```python
from build123d import *

# Parameters (mm, degrees)
SKETCH1_R               = 2
BOSS_EXTRUDE4_DEPTH     = 34.75
SKETCH5_R               = 2
CUT_EXTRUDE2_DEPTH      = 22.75
CUT_EXTRUDE3_REACH      = 59.871
CUT_EXTRUDE4_DEPTH      = 63.586120666
CUT_EXTRUDE5_REACH      = 61.819
CUT_EXTRUDE5_END_RADIUS = 37.906002519
SKETCH10_R              = 1.8
CUT_EXTRUDE6_REACH      = 59.074
SKETCH11_RX             = 1.8
SKETCH11_RY             = 1.799979565
CUT_EXTRUDE7_REACH      = 59.075
SKETCH11_4_RX           = 1.8
SKETCH11_4_RY           = 1.799979565
CUT_EXTRUDE8_DEPTH      = 9.85
SKETCH15_R              = 2
CUT_EXTRUDE9_DEPTH      = 2.38
SKETCH16_R              = 1.25
CUT_EXTRUDE10_DEPTH     = 6.1
SKETCH17_W              = 2.2
SKETCH17_H              = 4.33
CUT_EXTRUDE11_DEPTH     = 6.55
BOSS_EXTRUDE5_DEPTH     = 2.2
BOSS_EXTRUDE6_DEPTH     = 2.2


with BuildPart() as part:
    # Sketch1 → Boss-Extrude4 (new body)
    with BuildSketch(Plane.XY):
        with BuildLine():
            Line((-25.9, -19.75), (-11.5, -19.75))
            ThreePointArc((-11.5, -19.75), (-8.671572875, -18.578427125), (-7.5, -15.75))
            Line((-7.5, -15.75), (-7.5, -13))
            ThreePointArc((-7.5, -13), (0, -5.5), (7.5, -13))
            Line((7.5, -13), (7.5, -15.75))
            ThreePointArc((7.5, -15.75), (8.671572875, -18.578427125), (11.5, -19.75))
            Line((11.5, -19.75), (25.9, -19.75))
            ThreePointArc((25.9, -19.75), (31.556854249, -17.406854249), (33.9, -11.75))
            Line((33.9, -11.75), (33.9, 11.75))
            ThreePointArc((33.9, 11.75), (31.556854249, 17.406854249), (25.9, 19.75))
            Line((25.9, 19.75), (14.643684646, 19.75))
            ThreePointArc((14.643684646, 19.75), (0, 31.5), (-14.643684646, 19.75))
            Line((-14.643684646, 19.75), (-25.9, 19.75))
            ThreePointArc((-25.9, 19.75), (-31.556854249, 17.406854249), (-33.9, 11.75))
            Line((-33.9, 11.75), (-33.9, -11.75))
            ThreePointArc((-33.9, -11.75), (-31.556854249, -17.406854249), (-25.9, -19.75))
        make_face()
        with Locations((-15.9, 10.944699181)):
            Circle(SKETCH1_R, mode=Mode.SUBTRACT)
        with Locations(Location((-15.9, -10.944699181, 0), (0, 0, 180))):
            Circle(SKETCH1_R, mode=Mode.SUBTRACT)
        with Locations((15.9, -10.944699181)):
            Circle(SKETCH1_R, mode=Mode.SUBTRACT)
        with Locations(Location((15.9, 10.944699181, 0), (0, 0, 180))):
            Circle(SKETCH1_R, mode=Mode.SUBTRACT)
    extrude(amount=BOSS_EXTRUDE4_DEPTH)

    # Sketch5 → Cut-Extrude2 (cut)
    with BuildSketch(Plane.XY.offset(34.75)):
        with BuildLine():
            Line((33.9, -11.75), (33.9, 11.75))
            ThreePointArc((33.9, 11.75), (31.556854249, 17.406854249), (25.9, 19.75))
            Line((25.9, 19.75), (14.643684646, 19.75))
            ThreePointArc((14.643684646, 19.75), (0, 31.5), (-14.643684646, 19.75))
            Line((-14.643684646, 19.75), (-25.9, 19.75))
            ThreePointArc((-25.9, 19.75), (-31.556854249, 17.406854249), (-33.9, 11.75))
            Line((-33.9, 11.75), (-33.9, -11.75))
            ThreePointArc((-33.9, -11.75), (-31.556854249, -17.406854249), (-25.9, -19.75))
            Line((-25.9, -19.75), (-11.5, -19.75))
            ThreePointArc((-11.5, -19.75), (-8.671572875, -18.578427125), (-7.5, -15.75))
            Line((-7.5, -15.75), (-7.5, -13))
            ThreePointArc((-7.5, -13), (0, -5.5), (7.5, -13))
            Line((7.5, -13), (7.5, -15.75))
            ThreePointArc((7.5, -15.75), (8.671572875, -18.578427125), (11.5, -19.75))
            Line((11.5, -19.75), (25.9, -19.75))
            ThreePointArc((25.9, -19.75), (31.556854249, -17.406854249), (33.9, -11.75))
        make_face()
        with Locations((-15.9, 10.944699181)):
            Circle(SKETCH5_R, mode=Mode.SUBTRACT)
        with BuildLine():
            Line((-23.3, -3.45), (-23.3, 2.199999619))
            ThreePointArc((-23.3, 2.199999619), (0.199916465, 10.363760615), (23.699998093, 2.200475068))
            Line((23.699998093, 2.200475068), (23.699998093, -3.45))
            Line((23.699998093, -3.45), (-23.3, -3.45))
        make_face(mode=Mode.SUBTRACT)
    extrude(amount=-CUT_EXTRUDE2_DEPTH, mode=Mode.SUBTRACT)

    # Sketch6 → Cut-Extrude3 (cut, up to next)
    with BuildSketch(Plane.XY.offset(34.75), mode=Mode.PRIVATE) as cut_extrude3_sk1:
        with BuildLine():
            Line((-5.499999046, 14.493093188), (-5.499999046, 17.489830849))
            ThreePointArc((-5.499999046, 17.489830849), (0, 22.989829895), (5.499999046, 17.489830849))
            Line((5.499999046, 17.489830849), (5.499999046, 14.493093188))
            ThreePointArc((5.499999046, 14.493093188), (0, 8.993094142), (-5.499999046, 14.493093188))
        make_face()
    cut_extrude3_tool1 = extrude(cut_extrude3_sk1.sketch, amount=-CUT_EXTRUDE3_REACH, mode=Mode.PRIVATE) & part.part
    add(cut_extrude3_tool1.solids().sort_by_distance((0, 15.991462, 34.75))[0], mode=Mode.SUBTRACT)

    # Sketch9 → Cut-Extrude4 (cut, through all)
    with BuildSketch(Plane(origin=(0, 19.75, 0), x_dir=(1, 0, 0), z_dir=(0, 1, 0))):
        Polygon((-29.366805248, 0), (-26.65, -3.88), (-22.86, -3.88), (-20.143194752, 0), align=None)
        Polygon((22.86, -3.88), (20.143194752, 0), (29.366805248, 0), (26.65, -3.88), align=None)
    extrude(amount=-CUT_EXTRUDE4_DEPTH, mode=Mode.SUBTRACT)

    # Cut-Extrude5: up to this cylinder (the profile starts inside it)
    cut_extrude5_end = Plane(origin=(0.20029992, -27.542241902, 29.5), z_dir=(0, 0, 1)) * Cylinder(CUT_EXTRUDE5_END_RADIUS, 200.450005039, mode=Mode.PRIVATE)
    # Sketch10 → Cut-Extrude5 (cut, up to the surface)
    with BuildSketch(Plane.XZ.offset(3.45), mode=Mode.PRIVATE) as cut_extrude5_sk1:
        with Locations((-17.3, 29.5)):
            Circle(SKETCH10_R)
    cut_extrude5_tool1 = extrude(cut_extrude5_sk1.sketch, amount=-CUT_EXTRUDE5_REACH, mode=Mode.PRIVATE) & cut_extrude5_end
    add(cut_extrude5_tool1.solids().sort_by_distance((-17.3, -3.45, 29.5))[0], mode=Mode.SUBTRACT)
    # Sketch10 → Cut-Extrude5 (cut, up to the surface)
    with BuildSketch(Plane.XZ.offset(3.45), mode=Mode.PRIVATE) as cut_extrude5_sk2:
        with Locations((17.3, 29.5)):
            Circle(SKETCH10_R)
    cut_extrude5_tool2 = extrude(cut_extrude5_sk2.sketch, amount=-CUT_EXTRUDE5_REACH, mode=Mode.PRIVATE) & cut_extrude5_end
    add(cut_extrude5_tool2.solids().sort_by_distance((17.3, -3.45, 29.5))[0], mode=Mode.SUBTRACT)

    # Cut-Extrude6: up to this plane
    cut_extrude6_end = Plane(origin=(0, -1.1, 12), z_dir=(0, 1, 0))
    # Sketch11 → Cut-Extrude6 (cut, up to the surface)
    with BuildSketch(Plane(origin=(-0.04863224, 10.206057531, 0), x_dir=(-0.999988647405363, -0.004764982727443531, 0), z_dir=(0.00476498272744353, -0.9999886474053629, 0)), mode=Mode.PRIVATE) as cut_extrude6_sk1:
        Polygon((13.863688181, -29.5), (15.589965486, -32.49), (19.042520095, -32.49), (20.7687974, -29.5), (19.042520095, -26.51), (15.589965486, -26.51), align=None)
        with Locations(Location((17.316242791, -29.5), (0, 0, -90))):
            Ellipse(SKETCH11_RX, SKETCH11_RY, mode=Mode.SUBTRACT)
    cut_extrude6_tool1 = split(extrude(cut_extrude6_sk1.sketch, amount=CUT_EXTRUDE6_REACH, mode=Mode.PRIVATE), bisect_by=cut_extrude6_end, keep=Keep.BOTH, mode=Mode.PRIVATE)
    add(cut_extrude6_tool1.solids().sort_by_distance((-14.854399, 10.135508, 30.949327))[0], mode=Mode.SUBTRACT)
    # Sketch11 → Cut-Extrude6 (cut, up to the surface)
    with BuildSketch(Plane(origin=(-0.04863224, 10.206057531, 0), x_dir=(-0.999988647405363, -0.004764982727443531, 0), z_dir=(0.00476498272744353, -0.9999886474053629, 0)), mode=Mode.PRIVATE) as cut_extrude6_sk2:
        with Locations(Location((17.316242791, -29.5), (0, 0, -90))):
            Ellipse(SKETCH11_RX, SKETCH11_RY)
    cut_extrude6_tool2 = split(extrude(cut_extrude6_sk2.sketch, amount=CUT_EXTRUDE6_REACH, mode=Mode.PRIVATE), bisect_by=cut_extrude6_end, keep=Keep.BOTH, mode=Mode.PRIVATE)
    add(cut_extrude6_tool2.solids().sort_by_distance((-17.364678, 10.123546, 29.5))[0], mode=Mode.SUBTRACT)

    # Cut-Extrude7: up to this plane
    cut_extrude7_end = Plane(origin=(0, -1.1, 12), z_dir=(0, 1, 0))
    # Sketch11<4> → Cut-Extrude7 (cut, up to the surface)
    with BuildSketch(Plane(origin=(-0.04863224, 10.206057531, 0), x_dir=(-0.999988647405363, -0.004764982727443531, 0), z_dir=(0.00476498272744353, -0.9999886474053629, 0)), mode=Mode.PRIVATE) as cut_extrude7_sk1:
        Polygon((-13.8308098, -29.5), (-15.557087105, -26.51), (-19.009641715, -26.51), (-20.735919019, -29.5), (-19.009641715, -32.49), (-15.557087105, -32.49), align=None)
        with Locations(Location((-17.28336441, -29.5), (0, 0, -90))):
            Ellipse(SKETCH11_4_RX, SKETCH11_4_RY, mode=Mode.SUBTRACT)
    cut_extrude7_tool1 = split(extrude(cut_extrude7_sk1.sketch, amount=CUT_EXTRUDE7_REACH, dir=(0, -1, 0), mode=Mode.PRIVATE), bisect_by=cut_extrude7_end, keep=Keep.BOTH, mode=Mode.PRIVATE)
    add(cut_extrude7_tool1.solids().sort_by_distance((14.724256, 10.276451, 28.050673))[0], mode=Mode.SUBTRACT)
    # Sketch11<4> → Cut-Extrude7 (cut, up to the surface)
    with BuildSketch(Plane(origin=(-0.04863224, 10.206057531, 0), x_dir=(-0.999988647405363, -0.004764982727443531, 0), z_dir=(0.00476498272744353, -0.9999886474053629, 0)), mode=Mode.PRIVATE) as cut_extrude7_sk2:
        with Locations(Location((-17.28336441, -29.5), (0, 0, -90))):
            Ellipse(SKETCH11_4_RX, SKETCH11_4_RY)
    cut_extrude7_tool2 = split(extrude(cut_extrude7_sk2.sketch, amount=CUT_EXTRUDE7_REACH, dir=(0, -1, 0), mode=Mode.PRIVATE), bisect_by=cut_extrude7_end, keep=Keep.BOTH, mode=Mode.PRIVATE)
    add(cut_extrude7_tool2.solids().sort_by_distance((17.234536, 10.288412, 29.5))[0], mode=Mode.SUBTRACT)

    # Sketch14 → Cut-Extrude8 (cut)
    with BuildSketch(Plane(origin=(0, 0, 0), x_dir=(-1, 0, 0), z_dir=(0, 0, -1))):
        Polygon((0, 3), (9.959292144, 8.75), (9.959292144, 23.25), (0, 29), (-9.959292144, 23.25), (-9.959292144, 8.75), align=None)
    extrude(amount=-CUT_EXTRUDE8_DEPTH, mode=Mode.SUBTRACT)

    # Sketch15 → Cut-Extrude9 (cut)
    with BuildSketch(Plane.XY.offset(12)):
        Polygon((-14.167949192, 7.944699181), (-12.435898385, 10.944699181), (-14.167949192, 13.944699181), (-17.632050808, 13.944699181), (-19.364101615, 10.944699181), (-17.632050808, 7.944699181), align=None)
        with Locations((-15.9, 10.944699181)):
            Circle(SKETCH15_R, mode=Mode.SUBTRACT)
        with Locations((-15.9, 10.944699181)):
            Circle(SKETCH15_R)
        Polygon((14.167949192, 13.944699181), (17.632050808, 13.944699181), (19.364101615, 10.944699181), (17.632050808, 7.944699181), (14.167949192, 7.944699181), (12.435898385, 10.944699181), align=None)
        with Locations(Location((15.9, 10.944699181, 0), (0, 0, 180))):
            Circle(SKETCH15_R, mode=Mode.SUBTRACT)
        with Locations(Location((15.9, 10.944699181, 0), (0, 0, 180))):
            Circle(SKETCH15_R)
        Polygon((12.435898385, -10.944699181), (14.167949192, -13.944699181), (17.632050808, -13.944699181), (19.364101615, -10.944699181), (17.632050808, -7.944699181), (14.167949192, -7.944699181), align=None)
        with Locations((15.9, -10.944699181)):
            Circle(SKETCH15_R, mode=Mode.SUBTRACT)
        with Locations((15.9, -10.944699181)):
            Circle(SKETCH15_R)
        Polygon((-17.632050808, -13.944699181), (-19.364101615, -10.944699181), (-17.632050808, -7.944699181), (-14.167949192, -7.944699181), (-12.435898385, -10.944699181), (-14.167949192, -13.944699181), align=None)
        with Locations(Location((-15.9, -10.944699181, 0), (0, 0, 180))):
            Circle(SKETCH15_R, mode=Mode.SUBTRACT)
        with Locations(Location((-15.9, -10.944699181, 0), (0, 0, 180))):
            Circle(SKETCH15_R)
    extrude(amount=-CUT_EXTRUDE9_DEPTH, mode=Mode.SUBTRACT)

    # Sketch16 → Cut-Extrude10 (cut)
    with BuildSketch(Plane.ZY.offset(33.9)):
        with Locations((8.05, 1.13)):
            Circle(SKETCH16_R)
        with Locations((8.05, -8.33)):
            Circle(SKETCH16_R)
    extrude(amount=-CUT_EXTRUDE10_DEPTH, mode=Mode.SUBTRACT)

    # Sketch17 → Cut-Extrude11 (cut)
    with BuildSketch(Plane.XY.offset(12)):
        with Locations((-30.7, 1.13)):
            Rectangle(SKETCH17_W, SKETCH17_H)
        with Locations((-30.7, -8.33)):
            Rectangle(SKETCH17_W, SKETCH17_H)
    extrude(amount=-CUT_EXTRUDE11_DEPTH, mode=Mode.SUBTRACT)

    # Sketch18 → Boss-Extrude5 (add)
    with BuildSketch(Plane.ZY.offset(29.6)):
        Polygon((5.45, 3.295), (5.45, 1.13), (6.699963333, 3.295), align=None)
        Polygon((5.45, -1.035), (6.699963333, -1.035), (5.45, 1.13), align=None)
    extrude(amount=BOSS_EXTRUDE5_DEPTH)

    # Sketch21 → Boss-Extrude6 (add)
    with BuildSketch(Plane(origin=(-31.8, 0, 0), x_dir=(0, 0, -1), z_dir=(1, 0, 0))):
        Polygon((-5.45, -6.165), (-6.699963333, -6.165), (-5.45, -8.33), align=None)
        Polygon((-5.45, -10.495), (-5.45, -8.33), (-6.699963333, -10.495), align=None)
    extrude(amount=BOSS_EXTRUDE6_DEPTH)


solid = part.part
```
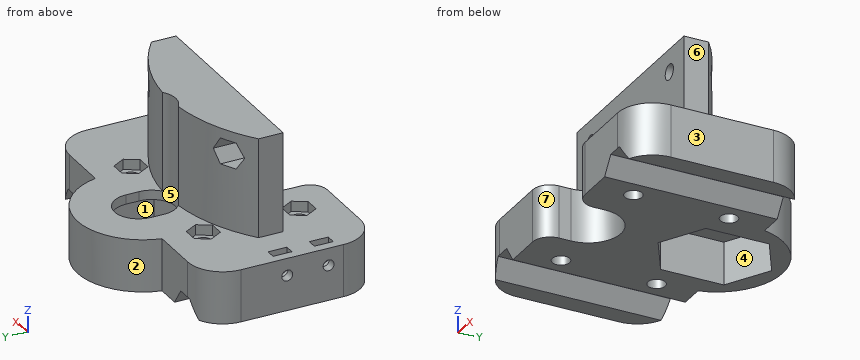
CAD build for the part. Positions are in the model's coordinates, mm. Face numbers are marked on the shaded views. A direction names the side the tool comes from. Round coordinates to 2 decimals unless told otherwise and drop trailing zeros. Write each loop counter-clockwise with the first axis right and the second up, starting at its lowest first coordinate (ties: lowest second). Pieces come first, ordered by that corner, then holes. Notation, with made-up numbers: (-28, 61.25) - (27, 61.25) arc R20 ccw to (27, 90.25) - close; hole circle Ø11 at (-10.75, 30.25). An arc over 180 degrees is marked (long way). Write item = value, one per line. Start each with the question number.
Q1. Band-saw the part on C-C (z = 18). Give the cut face in (x, y).
Q2. Band-saw the part on D-D (x = 6.5). Give the cut face in (y, z).
Q3. Drop flat-ended pins along their axis: pin 1 (5 mm diameter, centred on x = 5.5, y = 22.5, fed in from +Z); pin 2 (6 mm diameter, centred on y = 15, z = 14.5, fed in from +X); pin 3 (10 mm diameter, centred on x = 3.5, y = 13, fed in from -Z); pin 4 (10 mm diameter, centred on y = 19, z = 21, fed in from +X). Give the stop position or say it passes through.
Q4. Which spindle directions (+Z, -Z, +X, -X, +Y, -Y) get a long thin tool onto all of the face, cutting with end or side? Do the marked faces 4, 5, 6 and 7. Say none if no direction does.
Q5. Band-saw the part on A-A (x = -1). Give the cut face in (y, z).
Q6. Band-saw the part on B-B (z = 28.5). Give the cut face in (x, y).
Q7. Mould opens along X. For the marked faces 1, 2 and 3 say: pulls with the +X half, pulls with the -X half, needs draft (parallel to the pull), parting line crosses it, or undercut.
Q8. Probe L1, parallel to Y at x = -15.9, z = 3; L2, parallel to X at y = -10, z = 8.5; L3, parallel to Y at x = -33, z = 8. List the from-to ranges inside material, lowest first. Write a range as from..to.
Answers below:
q1.outline = (-23.3, -3.45) - (23.7, -3.45) - (23.7, 2.2) arc R37.91 ccw to (3.47, 10.22) arc R5.5 cw to (-3.43, 10.19) arc R37.91 ccw to (-23.3, 2.2) - close
q2.outline = (-9.26, 0) - (6.75, 0) - (6.75, 9.85) - (25.25, 9.85) - (25.25, 0) - (30.02, 0) - (30.02, 12) - (9.84, 12) - (9.84, 34.75) - (-3.45, 34.75) - (-3.45, 12) - (-9.26, 12) - close
q3.pin_1 = 12
q3.pin_2 = 33.74
q3.pin_3 = 9.85
q3.pin_4 = through
q4.face_4 = -Z
q4.face_5 = +Z, -Z
q4.face_6 = +Z, +X, +Y, -Y
q4.face_7 = +Z, -Z, -Y
q5.outline = (-5.57, 0) - (3.58, 0) - (3.58, 9.85) - (9.08, 9.85) - (9.08, 34.75) - (-3.45, 34.75) - (-3.45, 12) - (-5.57, 12) - close; (22.9, 9.85) - (28.42, 9.85) - (28.42, 0) - (31.47, 0) - (31.47, 12) - (22.9, 12) - close
q6.outline = (-23.3, -3.45) - (-18.8, -3.45) - (-18.8, -1.1) - (-20.19, -1.1) - (-20.21, 4.4) arc R37.91 ccw to (-23.3, 2.2) - close; (-15.8, -3.45) - (15.8, -3.45) - (15.8, -1.1) - (14.36, -1.1) - (14.36, 7.62) arc R37.91 ccw to (3.47, 10.22) arc R5.5 cw to (-3.43, 10.19) arc R37.91 ccw to (-14.48, 7.41) - (-14.44, -1.1) - (-15.8, -1.1) - close; (18.8, -3.45) - (23.7, -3.45) - (23.7, 2.2) arc R37.91 ccw to (20.11, 4.71) - (20.11, -1.1) - (18.8, -1.1) - close
q7.face_1 = undercut
q7.face_2 = parting line crosses it
q7.face_3 = pulls with the +X half
q8.L1 = -19.75..-12.94, -8.94..8.94, 12.94..19.75
q8.L2 = -33.9..-31.8, -29.6..-17.66, -14.14..-6.87, 6.87..14.14, 17.66..33.9
q8.L3 = -15.44..-9.58, -7.08..-0.12, 2.38..15.44
